Can you work these out from the model? Positions are in its coordinate system, mm. A direction names the side the tool comes from. Coordinates: 2 decimals unless noted, no trailing zeros. Put each result on its own line as item: value. Start each with the question number.
Item 1: For faces 1 (the cylindrical face through (1.43, 2.75, -2.25)), 2 (the flat face through (-0.1, -3.3, -2)), which set-ups out of +Z, -Z, +X, -X, +Y, -Y let a thin tool reach every point of the face, with its end or its side?
Item 2: Will these pins go through, and if not, where does the flat tip stop? P1, Ø5.5, axis at x = 0, y = 0, coming from the -Z side; P2, Ø1.5, axis at x = -3, z = 1, coming from the -Y side; P3, Ø3, axis at x = -1, y = 1.5, coming from the +Z side.
Item 3: Please list where these lines run through material, in increasing order: L1, parallel to Z at x = 2.25, y = 4.25; L2, parallel to X at y = 0, z = -2.2; L3, parallel to X at y = 0.75, z = -1.8. Write a range as from..to.
```python
from build123d import *

# Parameters (mm, degrees)
FILLET_R           = 0.5
SKETCH002_R        = 5
POCKET_DEPTH       = 4.5
SKETCH003_R        = 3.1
POCKET008003_DEPTH = 5.001


with BuildPart() as fillet_body:
    # Sketch001 → Revolution (revolve)
    with BuildSketch(Plane.XZ):
        Polygon((0, -2.5), (5.8, -2.5), (6.8, -1.5), (5.8, -0.5), (5.8, 0), (0, 0), align=None)
    revolve(axis=Axis((0, 0, 0), (0, 0, 1)))

    # Fillet
    fillet_edges = [fillet_body.edges().sort_by_distance(p)[0] for p in [
        (-6.8, 0, -1.5),
    ]]
    fillet(fillet_edges, radius=FILLET_R)


with BuildPart() as part_mirroring:
    # Part__Mirroring: instance of Fillet body
    add(fillet_body.part.mirror(Plane(origin=(0, 0, 0), x_dir=(0, 1, 0), z_dir=(0, 0, 1))))


with BuildPart() as bolthead001:
    # Fusion base: copy of Fillet body
    add(fillet_body.part)

    # Fusion: union Part__Mirroring
    add(part_mirroring.part)

    # Sketch002 → Pocket (cut)
    with BuildSketch(Plane.XY.offset(2.5)):
        Circle(SKETCH002_R)
    extrude(amount=-POCKET_DEPTH, mode=Mode.SUBTRACT)

    # Sketch003 → Pocket008003 (cut, through all)
    with BuildSketch(Plane(origin=(0, 0, -2.5), x_dir=(1, 0, 0), z_dir=(0, 0, -1))):
        Circle(SKETCH003_R)
    extrude(amount=-POCKET008003_DEPTH, mode=Mode.SUBTRACT)


solid = bolthead001.part
```
Solutions:
1. face 1: +Z, -Z
1. face 2: +Z
2. P1: through
2. P2: y = -6.14
2. P3: z = -2
3. L1: -2.5..-2
3. L2: -6.1..-3.1, 3.1..6.1
3. L3: -6.45..-4.94, 4.94..6.45
